Could you check a few things on this drawing? It's one solid part, dimensions in mm from its lowest x, y, z. A direction names the side the tool comes from. Round coordinates to 2 decimals unless told otherwise and drop trailing zeros. Write each loop counter-clockwise with the first axis right and the second up, starting at its lowest first coordinate (ties: lowest second). Pieces come first, ordered by that corner, then holes. Notation, with made-up numbers: (62, 21.25) -> (77, 21.25) arc R5 cw to (77, 28.25) -> close; hole circle Ø9 at (33, -18.75). An arc over 180 degrees is marked (long way). Answer in a Markdown table with one row per item. Add a question column.
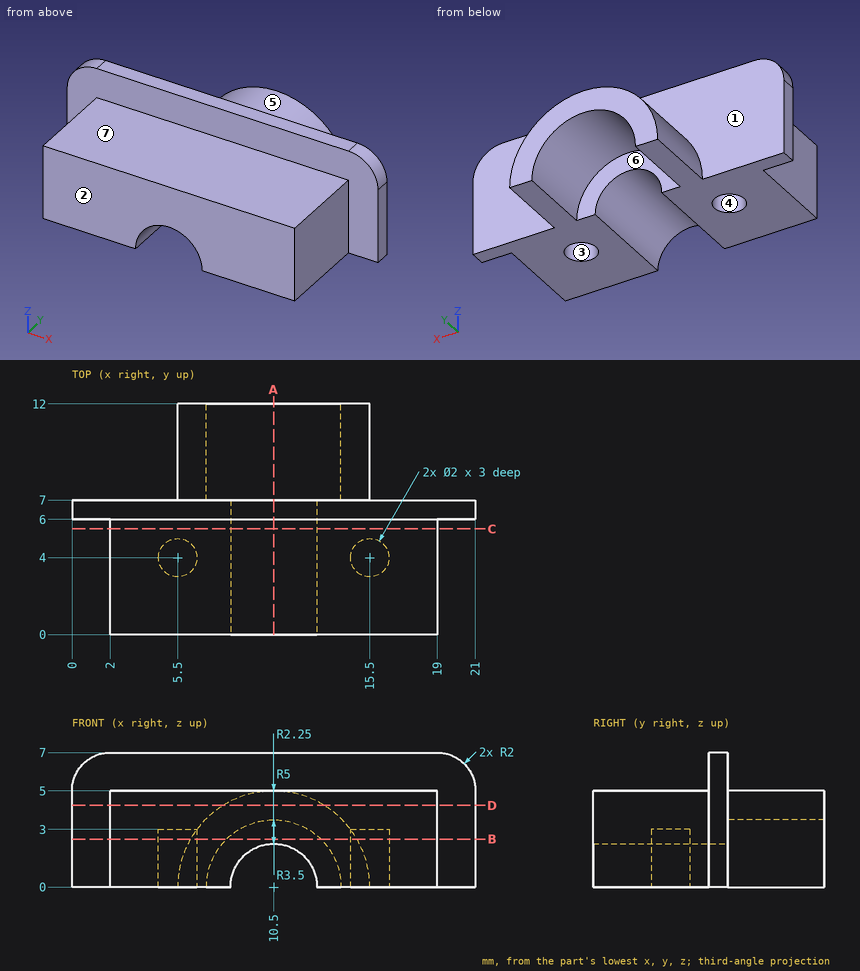
(1) Suppose I cut it at B-B, the plane z = 2.5. Please give me the cut outline in (x, y).
(2) Suppose I cut it at A-A, the plane x = 10.5. Please give me the cut outline in (y, z), then the cut area to 4 significant figures.
(3) Suppose I cut it at D-D, the plane z = 4.25. Please give me the cut outline in (x, y).
(4) Suppose I cut it at C-C, the plane y = 5.5. Please give me the cut outline in (x, z).
(5) On a 3-axis mill with a long thin cutter (end or side, diameter ignored), from which of +Z, -Z, +X, -X, +Y, -Y can I reach the whole of each face in a straight line? I mean the marked faces 4, 5, 6 and 7. Say none if no direction works.
(6) For P1, Ø2.5, axis at y = 3.5, z = 2.5, coming from the +X side; P2, Ø1.6, axis at x = 15.5, y = 4, coming from the +Z side; P3, Ø4, axis at x = 11.5, z = 1, coming from the +Y side, each with a flat end and sliding along its axis, tell me the tip position at first contact or that it passes through.
(7) If we mould it in two halves opening along Y, with no side actions, what happens to the marked faces 1, 2 and 3? For each: pulls with the +Y half, pulls with the -Y half, needs draft (parallel to the pull), parting line crosses it, or undercut.
(8) I need wall thicknesses on L1, parallel to Y at x = 5.5, z = 2.2; L2, parallel to Y at x = 19.25, z = 1.75; L3, parallel to Z at x = 17.75, y = 1.5. Which ranges of each line are inside material? Lowest first, please.
Response:
| question | item | result |
|---|---|---|
| 1 | outline | (0, 6) -> (2, 6) -> (2, 0) -> (19, 0) -> (19, 6) -> (21, 6) -> (21, 7) -> (14.83, 7) -> (14.83, 12) -> (12.95, 12) -> (12.95, 7) -> (8.05, 7) -> (8.05, 12) -> (6.17, 12) -> (6.17, 7) -> (0, 7) -> close; hole circle Ø2 at (5.5, 4); hole circle Ø2 at (15.5, 4) |
| 2 | outline | (0, 2.25) -> (7, 2.25) -> (7, 3.5) -> (12, 3.5) -> (12, 5) -> (7, 5) -> (7, 7) -> (6, 7) -> (6, 5) -> (0, 5) -> close |
| 2 | area | 28.75 mm² |
| 3 | outline | (0, 6) -> (2, 6) -> (2, 0) -> (19, 0) -> (19, 6) -> (21, 6) -> (21, 7) -> (13.13, 7) -> (13.13, 12) -> (7.87, 12) -> (7.87, 7) -> (0, 7) -> close |
| 4 | outline | (2, 0) -> (8.25, 0) arc R2.25 cw to (12.75, 0) -> (19, 0) -> (19, 5) -> (2, 5) -> close |
| 5 | face 4 | -Z |
| 5 | face 5 | +Z, +Y |
| 5 | face 6 | -Z, +Y |
| 5 | face 7 | +Z, +X, -X, -Y |
| 6 | P1 | x = 19 |
| 6 | P2 | z = 5 |
| 6 | P3 | y = 7 |
| 7 | face 1 | pulls with the +Y half |
| 7 | face 2 | pulls with the -Y half |
| 7 | face 3 | undercut |
| 8 | L1 | 0 to 3, 5 to 7 |
| 8 | L2 | 6 to 7 |
| 8 | L3 | 0 to 5 |
